CAD build for the part. Positions are in the model's coordinates, mm. Face numbers are marked on the shaded views. A direction names the side the tool comes from. Give positions to 0.01 mm unless a question says otherwise; leave off trailing zeros. Write each loop counter-clockwise with the first axis right and the second up, starting at its lowest first coordinate (ties: lowest second). Pieces come first, ordered by that corner, then holes. Notation, with made-up numbers: (19, 72) -> (27, 72) arc R31 ccw to (27, 111) -> close; hole circle Ø6 at (-37, -32.75). An arc over 180 degrees is marked (long way). Answer as a JSON object with one key per item and string values.
```python
from build123d import *

# Parameters (mm, degrees)
F0_W      = 260.35
F0_H      = 9.525
F1_DEPTH  = 76.2
F2_W      = 260.35
F2_H      = 152.4
F2_W_2    = 241.3
F2_H_2    = 133.35
F3_DEPTH  = 44.45
F5_DEPTH  = 44.45
F7_DEPTH  = 88.9
F9_DEPTH  = 12.7
F11_DEPTH = 223.52


with BuildPart() as f1:
    # F0 (on Front) → F1 (new body, symmetric)
    with BuildSketch(Plane.XZ):
        with Locations((0, 4.7625)):
            Rectangle(F0_W, F0_H)
    extrude(amount=F1_DEPTH, both=True)

    # F2 (on face) → F3 (join)
    with BuildSketch(Plane.XY.offset(9.525)):
        Rectangle(F2_W, F2_H)
        Rectangle(F2_W_2, F2_H_2, mode=Mode.SUBTRACT)
    extrude(amount=F3_DEPTH)

    # F4 (on face) → F5 (join)
    with BuildSketch(Plane.XY.offset(9.525)):
        Polygon((-4.7625, -66.675), (0, -66.675), (4.7625, -66.675), (4.7625, 66.675), (0, 66.675), (-4.7625, 66.675), align=None)
    extrude(amount=F5_DEPTH)

    # F6 (on face) → F7 (join)
    with BuildSketch(Plane.XY.offset(9.525)):
        Polygon((-120.65, 6.35), (-120.65, 0), (-120.65, -6.35), (120.65, -6.35), (120.65, 6.35), align=None)
    extrude(amount=F7_DEPTH)

    # F8 (on face) → F9 (cut)
    with BuildSketch(Plane.XZ.offset(6.35)):
        with BuildLine():
            ThreePointArc((24.1451865613, 57.15), (36.8451865613, 69.85), (24.1451865613, 82.55))
            Line((24.1451865613, 82.55), (-26.6548134387, 82.55))
            ThreePointArc((-26.6548134387, 82.55), (-39.3548134387, 69.85), (-26.6548134387, 57.15))
            Line((-26.6548134387, 57.15), (24.1451865613, 57.15))
        make_face()
    extrude(amount=-F9_DEPTH, mode=Mode.SUBTRACT)

    # F10 (on face) → F11 (cut)
    with BuildSketch(Plane.XZ.offset(76.2)):
        with BuildLine():
            ThreePointArc((0, 247.2596246621), (-267.4707294697, 311.9378914894), (-149.1386400133, 63.5))
            ThreePointArc((-149.1386400133, 63.5), (-53.1007485209, 97.5679105219), (0, 184.5403753379))
            ThreePointArc((0, 184.5403753379), (-3.26136, 215.9), (0, 247.2596246621))
        make_face()
        with BuildLine():
            ThreePointArc((0, 247.2596246621), (-3.26136, 215.9), (0, 184.5403753379))
            ThreePointArc((0, 184.5403753379), (2.4438272183, 200.1356214204), (3.26136, 215.9))
            ThreePointArc((3.26136, 215.9), (2.4438272183, 231.6643785796), (0, 247.2596246621))
        make_face()
        with BuildLine():
            ThreePointArc((0, 184.5403753379), (53.1007485157, 97.5679105261), (149.13864, 63.5))
            ThreePointArc((149.13864, 63.5), (256.9017134528, 108.1369265472), (301.53864, 215.9))
            ThreePointArc((301.53864, 215.9), (164.9030185796, 367.4824672183), (0, 247.2596246621))
            ThreePointArc((0, 247.2596246621), (2.4438272183, 231.6643785796), (3.26136, 215.9))
            ThreePointArc((3.26136, 215.9), (2.4438272183, 200.1356214204), (0, 184.5403753379))
        make_face()
    extrude(amount=-F11_DEPTH, mode=Mode.SUBTRACT)


solid = f1.part
```
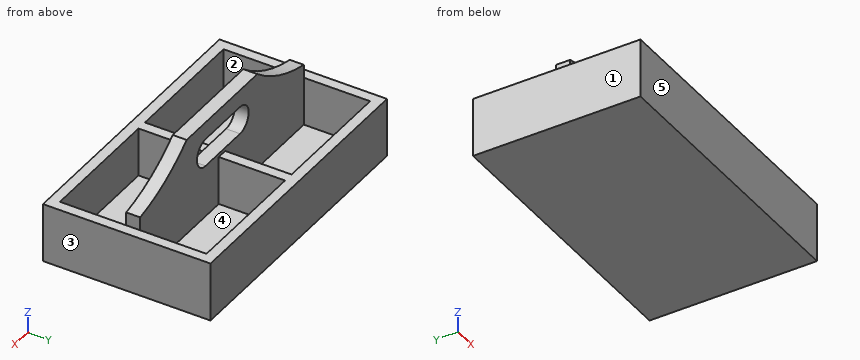
1) Slice it at C-C (z = 38). State how many separate pieces and enclosed holes the cut face has, then the cut area to 3 significant figures.
Model answer:
{"separate pieces": "1", "enclosed holes": "4", "area": "11,700 mm2"}
2) Wall check: probe 1 along Y at (x, z) = (-76, 28.5) (3 decimals); probe 2 along Y at (x, z) = (-82.5, 56). Give the ranges that are in metal, low to high.
Model answer:
{"probe 1": "y = -76.2 to -66.675, -6.35 to 6.35, 66.675 to 76.2", "probe 2": "y = -6.35 to 6.35"}
3) Pin check, flat tips, straight feed: pin 1 (1.5 mm diameter, centred on x = -56.5, y = 22, fed in from +Z) (3 decimals); pin 2 (6 mm diameter, centred on y = -0.5, z = 57.5, fed in from +X); pin 3 (10 mm diameter, centred on x = -69, z = 71, fed in from +Y). Stop position of each tip, or through.
Model answer:
{"pin 1": "stops at z = 9.525", "pin 2": "stops at x = 120.65", "pin 3": "stops at y = 6.35"}
4) 3-axis set-ups, long thin cutter, end or side, ignore diameter. For the marked faces 1 and 2: which of +Z, -Z, +X, -X, +Y, -Y reach the whole face in a straight line?
Model answer:
{"face 1": "+Z, -Z, -X, +Y, -Y", "face 2": "+Z"}
5) Slice it at A-A (x = 13). List the corners of the cut face in (y, z) (3 decimals), then the cut area to 3 significant figures.
Model answer:
{"outline": "(-76.2, 0) -> (76.2, 0) -> (76.2, 53.975) -> (66.675, 53.975) -> (66.675, 9.525) -> (6.35, 9.525) -> (6.35, 57.15) -> (-6.35, 57.15) -> (-6.35, 9.525) -> (-66.675, 9.525) -> (-66.675, 53.975) -> (-76.2, 53.975) -> close; (-6.35, 82.55) -> (6.35, 82.55) -> (6.35, 98.425) -> (-6.35, 98.425) -> close", "area": "3,100 mm2"}
6) Mould opens along Y. For the marked faces 3, 4 and 5 say: released by +Y, released by -Y, zero draft, split by the parting line, or undercut.
Model answer:
{"face 3": "zero draft", "face 4": "undercut", "face 5": "released by -Y"}
7) Slice it at D-D (z = 69.85). List the corners of the cut face in (x, y), then the cut area to 3 significant figures.
Model answer:
{"outline": "(-105.61, -6.35) -> (-39.35, -6.35) -> (-39.35, 6.35) -> (-105.61, 6.35) -> close; (36.85, -6.35) -> (105.61, -6.35) -> (105.61, 6.35) -> (36.85, 6.35) -> close", "area": "1,710 mm2"}
